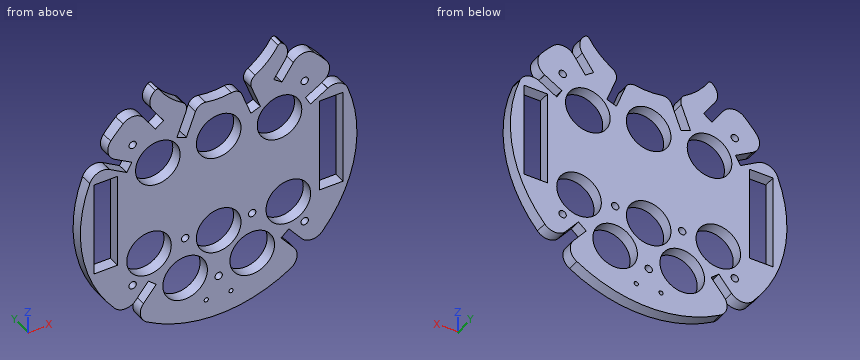
from build123d import *

# Parameters (mm, degrees)
SKETCH1_R           = 2
SKETCH1_W           = 12.7
SKETCH1_H           = 50.8
SKETCH1_R_2         = 12.095
SKETCH1_R_3         = 12.075
SKETCH1_R_4         = 1.143
BOSS_EXTRUDE1_DEPTH = 6.35


with BuildPart() as part:
    # Sketch1 → Boss-Extrude1 (new body)
    with BuildSketch(Plane(origin=(0, 0, 0), x_dir=(1, 0, 0), z_dir=(0, 1, 0))):
        with BuildLine():
            Line((-40.520093651, -53.074212293), (-34.358059191, -44.273915061))
            Line((-34.358059191, -44.273915061), (-29.852722948, -47.428585461))
            Line((-29.852722948, -47.428585461), (-36.014757408, -56.228882693))
            ThreePointArc((-36.014757408, -56.228882693), (-37.282182463, -61.682274385), (-34.419720881, -66.493943628))
            ThreePointArc((-34.419720881, -66.493943628), (-33.243515234, -66.777434912), (-32.240681933, -66.10056535))
            ThreePointArc((-32.240681933, -66.10056535), (-26.728650164, -59.250774979), (-19.793246149, -53.846860332))
            ThreePointArc((-19.793246149, -53.846860332), (-17.659799789, -51.192486841), (-17.721018114, -47.787557426))
            Line((-17.721018114, -47.787557426), (-22.618223277, -34.99005566))
            Line((-22.618223277, -34.99005566), (-17.481479686, -33.024383946))
            Line((-17.481479686, -33.024383946), (-12.584274523, -45.821885712))
            ThreePointArc((-12.584274523, -45.821885712), (-10.356790186, -48.397852623), (-6.996351286, -48.949887413))
            ThreePointArc((-6.996351286, -48.949887413), (0, -48.302004425), (6.996351286, -48.949887413))
            ThreePointArc((6.996351286, -48.949887413), (10.356790186, -48.397852623), (12.584274523, -45.821885712))
            Line((12.584274523, -45.821885712), (17.481479686, -33.024383946))
            Line((17.481479686, -33.024383946), (22.618223277, -34.99005566))
            Line((22.618223277, -34.99005566), (17.721018114, -47.787557426))
            ThreePointArc((17.721018114, -47.787557426), (17.659799789, -51.192486841), (19.793246149, -53.846860332))
            ThreePointArc((19.793246149, -53.846860332), (26.728650164, -59.250774979), (32.240681933, -66.10056535))
            ThreePointArc((32.240681933, -66.10056535), (33.243515234, -66.777434912), (34.419720881, -66.493943628))
            ThreePointArc((34.419720881, -66.493943628), (37.282182463, -61.682274385), (36.014757408, -56.228882693))
            Line((36.014757408, -56.228882693), (29.852722948, -47.428585461))
            Line((29.852722948, -47.428585461), (34.358059191, -44.273915061))
            Line((34.358059191, -44.273915061), (40.520093651, -53.074212293))
            ThreePointArc((40.520093651, -53.074212293), (45.927580176, -56.23617342), (51.848593315, -54.191543356))
            ThreePointArc((51.848593315, -54.191543356), (55.295899374, -50.669157408), (58.504414423, -46.927960674))
            ThreePointArc((58.504414423, -46.927960674), (60.030901261, -40.882046302), (56.458030011, -35.771485305))
            Line((56.458030011, -35.771485305), (56.349654942, -35.70891493))
            Line((56.349654942, -35.70891493), (47.078155187, -30.35601205))
            Line((47.078155187, -30.35601205), (49.828155187, -25.59287233))
            Line((49.828155187, -25.59287233), (59.099654942, -30.945775209))
            Line((59.099654942, -30.945775209), (59.208030011, -31.008345585))
            ThreePointArc((59.208030011, -31.008345585), (65.420341286, -31.547262353), (69.893013303, -27.202328787))
            ThreePointArc((69.893013303, -27.202328787), (73.860606951, 13.023468848), (56.374397975, 49.466425512))
            ThreePointArc((56.374397975, 49.466425512), (50.654117331, 52.01932544), (44.991624855, 49.340690033))
            Line((44.991624855, 49.340690033), (38.069871869, 41.091666046))
            Line((38.069871869, 41.091666046), (33.856627432, 44.626997899))
            Line((33.856627432, 44.626997899), (40.778380417, 52.876021886))
            ThreePointArc((40.778380417, 52.876021886), (42.433039833, 58.917628536), (38.925607882, 64.107698843))
            ThreePointArc((38.925607882, 64.107698843), (0, 75), (-38.925607882, 64.107698843))
            ThreePointArc((-38.925607882, 64.107698843), (-42.433039833, 58.917628536), (-40.778380417, 52.876021886))
            Line((-40.778380417, 52.876021886), (-33.856627432, 44.626997899))
            Line((-33.856627432, 44.626997899), (-38.069871869, 41.091666046))
            Line((-38.069871869, 41.091666046), (-44.991624855, 49.340690033))
            ThreePointArc((-44.991624855, 49.340690033), (-50.654117331, 52.01932544), (-56.374397975, 49.466425512))
            ThreePointArc((-56.374397975, 49.466425512), (-73.860606951, 13.023468848), (-69.893013303, -27.202328787))
            ThreePointArc((-69.893013303, -27.202328787), (-65.420341286, -31.547262353), (-59.208030011, -31.008345585))
            Line((-59.208030011, -31.008345585), (-59.099654942, -30.945775209))
            Line((-59.099654942, -30.945775209), (-49.828155187, -25.59287233))
            Line((-49.828155187, -25.59287233), (-47.078155187, -30.35601205))
            Line((-47.078155187, -30.35601205), (-56.349654942, -35.70891493))
            Line((-56.349654942, -35.70891493), (-56.458030011, -35.771485305))
            ThreePointArc((-56.458030011, -35.771485305), (-60.030901261, -40.882046302), (-58.504414423, -46.927960674))
            ThreePointArc((-58.504414423, -46.927960674), (-55.295899374, -50.669157408), (-51.848593315, -54.191543356))
            ThreePointArc((-51.848593315, -54.191543356), (-45.927580176, -56.23617342), (-40.520093651, -53.074212293))
        make_face()
        with Locations((-46.663733983, -40.081231883)):
            Circle(SKETCH1_R, mode=Mode.SUBTRACT)
        with Locations((-61.164123727, 0)):
            Rectangle(SKETCH1_W, SKETCH1_H, mode=Mode.SUBTRACT)
        with Locations((-32.995567884, -24.592872328)):
            Circle(SKETCH1_R_2, mode=Mode.SUBTRACT)
        with Locations((46.663733983, -40.081231883)):
            Circle(SKETCH1_R, mode=Mode.SUBTRACT)
        with Locations((0, -26.93833729)):
            Circle(SKETCH1_R_2, mode=Mode.SUBTRACT)
        with Locations((32.995567884, -24.592872328)):
            Circle(SKETCH1_R_2, mode=Mode.SUBTRACT)
        with Locations((61.164123727, 0)):
            Rectangle(SKETCH1_W, SKETCH1_H, mode=Mode.SUBTRACT)
        with Locations((-37.772386793, 25.4)):
            Circle(SKETCH1_R_3, mode=Mode.SUBTRACT)
        with Locations((-18.178952795, 24.310551096)):
            Circle(SKETCH1_R, mode=Mode.SUBTRACT)
        with Locations((-46.663733983, 40.081231883)):
            Circle(SKETCH1_R, mode=Mode.SUBTRACT)
        with Locations((-18.1962694, 47.045805056)):
            Circle(SKETCH1_R_2, mode=Mode.SUBTRACT)
        with Locations((-6.731, 64.107698843)):
            Circle(SKETCH1_R_4, mode=Mode.SUBTRACT)
        with Locations((0, 26.93833729)):
            Circle(SKETCH1_R_2, mode=Mode.SUBTRACT)
        with Locations((18.178952795, 24.310551096)):
            Circle(SKETCH1_R, mode=Mode.SUBTRACT)
        with Locations((37.772386793, 25.4)):
            Circle(SKETCH1_R_2, mode=Mode.SUBTRACT)
        with Locations((18.1962694, 47.045805056)):
            Circle(SKETCH1_R_2, mode=Mode.SUBTRACT)
        with Locations((0, 53.061187965)):
            Circle(SKETCH1_R, mode=Mode.SUBTRACT)
        with Locations((6.731, 64.107698843)):
            Circle(SKETCH1_R_4, mode=Mode.SUBTRACT)
        with Locations((46.663733983, 40.081231883)):
            Circle(SKETCH1_R, mode=Mode.SUBTRACT)
    extrude(amount=BOSS_EXTRUDE1_DEPTH)


solid = part.part
Build history of the part. All positions in model axes, mm. Round coordinates to 2 decimals unless told otherwise and drop trailing zeros. Write each loop counter-clockwise with the first axis right and the second up, starting at its lowest first coordinate (ties: lowest second). Pieces come first, ordered by that corner, then holes. Notation, with made-up numbers: M 55,-6 L 59,-6 A30 cw 59,19 Z; hole C 27,54 d6. An arc over 180 degrees is marked long. Answer as a JSON object with one key per item and string values. Group by question number.
(1) Drill centre lines: L1, parallel to X at y = 1, z = 1.5 (3 decimals); L2, parallel to Z at x = 0, y = 2.25; L3, parallel to X at y = 1, z = -4. Where is each one in solid material? Low to high.
(2) Flat gauge pins, fed straight in: pin 1 (3 mm diameter, centred on x = 16, y = 5, fed in from -Z) (3 decimals); pin 2 (5 mm diameter, centred on x = -46.66, z = 40.08, fed in from +Y); pin 3 (19.5 mm diameter, centred on x = -37.77, z = -25.4, fed in from +Y); pin 4 (1 mm diameter, centred on x = 57.5, y = 4, fed in from +Z). Where does each tip first touch, or does it go through?
(3) Cut at B-B (y = 2.5). Give the number of separate pieces and of enclosed holes in the cut face, and give its area (3 significant figures).
(4) Cut at A-A (x = 0). Give the cut face in (y, z), and give its area (3 significant figures).
Responses:
{
 "1": {"L1": "x = -74.985 to -67.514, -54.814 to 54.814, 67.514 to 74.985", "L2": "z = -75 to -55.06, -51.06 to -39.03, -14.84 to 14.84, 39.03 to 48.3", "L3": "x = -74.89 to -67.51, -54.81 to 54.81, 67.51 to 74.89"},
 "2": {"pin 1": "stops at z = -73.585", "pin 2": "stops at y = 6.35", "pin 3": "passes through", "pin 4": "stops at z = 48.74"},
 "3": {"separate pieces": "1", "enclosed holes": "19", "area": "10,300 mm2"},
 "4": {"outline": "M 0,-75 L 6.35,-75 L 6.35,-55.06 L 0,-55.06 Z; M 0,-51.06 L 6.35,-51.06 L 6.35,-39.03 L 0,-39.03 Z; M 0,-14.84 L 6.35,-14.84 L 6.35,14.84 L 0,14.84 Z; M 0,39.03 L 6.35,39.03 L 6.35,48.3 L 0,48.3 Z", "area": "450 mm2"}
}
